Read the model definition and answer for the solid it produces. Units are mm, in the model's axes. A direction names the side the tool comes from. Coordinates: 2 decimals unless noted, no trailing zeros. Write each loop counter-clockwise with the first axis right and the second up, starting at its lowest first coordinate (ties: lowest second). Pieces come first, ordered by that corner, then holes.
(1) Section D-D on x = 0 is taken. Write down the section's boundary in (y, z).
(2) Section A-A on z = 0 is taken. Write down the section's boundary in (x, y), then the cut area to 3 significant figures.
(3) Find the intervals of material crossed by probe 1 along Z at (x, y) = (0, 63); probe 2 along X at (y, z) = (62.65, 0); probe 3 along Y at (x, z) = (-22.5, -23), in increasing order.
(4) Section C-C on y = 28.5 is taken. Write down the section's boundary in (x, z).
(5) Given pin 1 (0.9 mm diameter, centred on y = 60, z = 13.5, fed in from +X); pin 2 (2 mm diameter, centred on x = 43.5, y = 10, fed in from +Z); pin 3 (8 mm diameter, centred on y = 44, z = 1, fed in from -X); pin 4 (8 mm diameter, centred on y = 35.5, z = -1, fed in from +X), each flat-ended and moving along its own axis, determine where each tip first touches the part or whether it passes through.
(6) Which of the six approach directions +Z, -Z, +X, -X, +Y, -Y give full straight-line access (tool end or side, diameter ignored) to faces 1 (the cylindrical face through (2.79, 63.54, -77.95)), 2 (the flat face through (60.661, 12.325, 36.594)), 3 (the flat face through (-30, 40, 56)), 4 (the cylindrical face through (32.66, 58.71, -30.74))?
(7) The mould has two halves that part along X. Classify faces 5 (the flat face through (-67, 0, 43)), 6 (the cylindrical face through (-62, 11, -58)), 7 (the flat face through (-30, 40, -55)): +X half, -X half, draft (parallel to the pull), parting line (faces both ways), or undercut.
(8) Section B-B on y = 19 is taken. Write down the section's boundary in (x, z).
from build123d import *

# Parameters (mm, degrees)
BOSS_EXTRUDE1_DEPTH     = 66
CUT_EXTRUDE3_DEPTH      = 25
CUT_EXTRUDE3_DEPTH_BACK = 10
FILLET1_R               = 4
FILLET3_R               = 9
SKETCH4_W               = 60
SKETCH4_H               = 150
CUT_EXTRUDE4_DEPTH      = 33
CUT_EXTRUDE5_DEPTH      = 5
CUT_EXTRUDE6_DEPTH      = 132.030530793
FILLET5_R               = 3
FILLET6_R               = 5
FILLET7_R               = 3
SKETCH7_R               = 1.5
CUT_EXTRUDE7_DEPTH      = 198.739948877
SKETCH11_R              = 3
CUT_EXTRUDE10_DEPTH     = 210.0771447
SKETCH8_R               = 1.5
CUT_EXTRUDE8_DEPTH      = 205.670582053
SKETCH10_R              = 3
CUT_EXTRUDE9_DEPTH      = 216.914390172
FILLET10_R              = 5


with BuildPart() as part:
    # Sketch3 → Boss-Extrude1 (new body)
    with BuildSketch(Plane(origin=(0, 0, 0), x_dir=(1, 0, 0), z_dir=(0, 1, 0))):
        with BuildLine():
            Line((-46.032597146, -75), (46.032597146, -75))
            ThreePointArc((46.032597146, -75), (0, 88), (-46.032597146, -75))
        make_face()
    extrude(amount=BOSS_EXTRUDE1_DEPTH)

    # Sketch2 → Cut-Extrude3 (cut, two sides: drawn at the far end of the back side and taken through both)
    with BuildSketch(Plane(origin=(0, 0, 0), x_dir=(1, 0, 0), z_dir=(0, 1, 0)).offset(-CUT_EXTRUDE3_DEPTH_BACK)):
        with BuildLine():
            Line((68.882903046, 31.406243643), (31.406243643, 68.882903046))
            Line((31.406243643, 68.882903046), (40.598631798, 78.075291201))
            ThreePointArc((40.598631798, 78.075291201), (0, 88), (-40.598631798, 78.075291201))
            Line((-40.598631798, 78.075291201), (-31.406243643, 68.882903046))
            Line((-31.406243643, 68.882903046), (-68.882903046, 31.406243643))
            Line((-68.882903046, 31.406243643), (-78.075291201, 40.598631798))
            ThreePointArc((-78.075291201, 40.598631798), (-87.22877857, 11.624981252), (-85.982636075, -18.734628196))
            Line((-85.982636075, -18.734628196), (-74.724305826, -12.234628196))
            Line((-74.724305826, -12.234628196), (-47.724305826, -59))
            Line((-47.724305826, -59), (-47.724305826, -73.935043338))
            ThreePointArc((-47.724305826, -73.935043338), (-46.881475519, -74.472325418), (-46.032597146, -75))
            ThreePointArc((-46.032597146, -75), (0, -88), (46.032597146, -75))
            ThreePointArc((46.032597146, -75), (46.881475519, -74.472325418), (47.724305826, -73.935043338))
            Line((47.724305826, -73.935043338), (47.724305826, -59))
            Line((47.724305826, -59), (74.724305826, -12.234628196))
            Line((74.724305826, -12.234628196), (85.982636075, -18.734628196))
            ThreePointArc((85.982636075, -18.734628196), (87.49420545, -9.421465529), (88, 0))
            ThreePointArc((88, 0), (85.482821741, 20.897061687), (78.075291201, 40.598631798))
            Line((78.075291201, 40.598631798), (68.882903046, 31.406243643))
        make_face()
    extrude(amount=CUT_EXTRUDE3_DEPTH + CUT_EXTRUDE3_DEPTH_BACK, mode=Mode.SUBTRACT)

    # Fillet1
    fillet1_edges = [part.edges().sort_by_distance(p)[0] for p in [
        (74.724305826, 12.5, 12.234628196),
        (68.882903046, 12.5, -31.406243643),
        (31.406243643, 12.5, -68.882903046),
        (-31.406243643, 12.5, -68.882903046),
        (-68.882903046, 12.5, -31.406243643),
        (-74.724305826, 12.5, 12.234628196),
    ]]
    fillet(fillet1_edges, radius=FILLET1_R)

    # Fillet3
    fillet3_edges = [part.edges().sort_by_distance(p)[0] for p in [
        (47.724305826, 12.5, 59),
        (-47.724305826, 12.5, 59),
    ]]
    fillet(fillet3_edges, radius=FILLET3_R)

    # Sketch4 → Cut-Extrude4 (cut)
    with BuildSketch(Plane.XZ.offset(-25)):
        Rectangle(SKETCH4_W, SKETCH4_H)
        with BuildLine():
            Line((30, -75), (-30, -75))
            ThreePointArc((-30, -75), (0, -80.777472107), (30, -75))
        make_face()
    extrude(amount=-CUT_EXTRUDE4_DEPTH, mode=Mode.SUBTRACT)

    # Sketch5 → Cut-Extrude5 (cut)
    with BuildSketch(Plane(origin=(0, 66, 0), x_dir=(1, 0, 0), z_dir=(0, 1, 0))):
        with BuildLine():
            Line((-43.116122275, -65), (43.116122275, -65))
            ThreePointArc((43.116122275, -65), (0, 78), (-43.116122275, -65))
        make_face()
    extrude(amount=-CUT_EXTRUDE5_DEPTH, mode=Mode.SUBTRACT)

    # Sketch6 → Cut-Extrude6 (cut, through all)
    with BuildSketch(Plane.XZ.offset(-25)):
        Polygon((30, 35), (50, 15), (50, -15), (30, -35), align=None)
        Polygon((-50, -15), (-30, -35), (-30, 35), (-50, 15), align=None)
    extrude(amount=-CUT_EXTRUDE6_DEPTH, mode=Mode.SUBTRACT)

    # Fillet5
    fillet5_edges = [part.edges().sort_by_distance(p)[0] for p in [
        (30, 59.5, -35),
        (30, 59.5, 35),
        (-30, 59.5, 35),
        (-30, 59.5, -35),
    ]]
    fillet(fillet5_edges, radius=FILLET5_R)

    # Fillet6
    fillet6_edges = [part.edges().sort_by_distance(p)[0] for p in [
        (30, 41.5, -35),
        (30, 41.5, 35),
        (50, 43, 15),
        (50, 43, -15),
        (-30, 41.5, 35),
        (-50, 43, -15),
        (-50, 43, 15),
        (-30, 41.5, -35),
    ]]
    fillet(fillet6_edges, radius=FILLET6_R)

    # Fillet7
    fillet7_edges = [part.edges().sort_by_distance(p)[0] for p in [
        (-30, 41.5, -75),
        (30, 58, -56.035533906),
        (0, 58, -80.777472107),
        (30, 41.5, -75),
        (-30, 58, -56.035533906),
        (-33.292893219, 58, 31.707106781),
        (33.292893219, 58, -31.707106781),
        (33.292893219, 58, 31.707106781),
        (30, 58, 56.035533906),
        (-30, 58, 56.035533906),
        (-33.292893219, 58, -31.707106781),
        (30.380602337, 58, -35.15765065),
        (30.380602337, 58, 35.15765065),
        (-30.380602337, 58, 35.15765065),
        (-30.380602337, 58, -35.15765065),
    ]]
    fillet(fillet7_edges, radius=FILLET7_R)

    # Sketch7 → Cut-Extrude7 (cut, through all)
    with BuildSketch(Plane(origin=(50.144573344, 0, -50.144573344), x_dir=(0.7071067811865472, 0, 0.7071067811865478), z_dir=(-0.7071067811865478, 0, 0.7071067811865472))):
        with Locations((0, 10)):
            Circle(SKETCH7_R)
    cut_extrude7 = extrude(amount=-CUT_EXTRUDE7_DEPTH, mode=Mode.SUBTRACT)

    # Sketch11 → Cut-Extrude10 (cut, through all)
    with BuildSketch(Plane(origin=(58.629854718, 0, -58.629854718), x_dir=(0.7071067811865472, 0, 0.7071067811865478), z_dir=(-0.7071067811865478, 0, 0.7071067811865472))):
        with Locations((0, 10)):
            Circle(SKETCH11_R)
    cut_extrude10 = extrude(amount=-CUT_EXTRUDE10_DEPTH, mode=Mode.SUBTRACT)

    # Sketch8 → Cut-Extrude8 (cut, through all)
    with BuildSketch(Plane(origin=(61.340978781, 0, 35.415230611), x_dir=(-0.5000000000000003, 0, 0.8660254037844386), z_dir=(-0.8660254037844385, 0, -0.5000000000000002))):
        with Locations((0, 10)):
            Circle(SKETCH8_R)
    cut_extrude8 = extrude(amount=-CUT_EXTRUDE8_DEPTH, mode=Mode.SUBTRACT)

    # Sketch10 → Cut-Extrude9 (cut, through all)
    with BuildSketch(Plane(origin=(71.733283626, 0, 41.415230611), x_dir=(-0.5000000000000003, 0, 0.8660254037844386), z_dir=(-0.8660254037844385, 0, -0.5000000000000002))):
        with Locations((0, 10)):
            Circle(SKETCH10_R)
    cut_extrude9 = extrude(amount=-CUT_EXTRUDE9_DEPTH, mode=Mode.SUBTRACT)

    # Mirror1: Cut-Extrude7, Cut-Extrude10, Cut-Extrude8, Cut-Extrude9 across plane
    add(cut_extrude7.mirror(Plane(origin=(0, 0, 0), x_dir=(0, 0, 1), z_dir=(1, 0, 0))), mode=Mode.SUBTRACT)
    add(cut_extrude10.mirror(Plane(origin=(0, 0, 0), x_dir=(0, 0, 1), z_dir=(1, 0, 0))), mode=Mode.SUBTRACT)
    add(cut_extrude8.mirror(Plane(origin=(0, 0, 0), x_dir=(0, 0, 1), z_dir=(1, 0, 0))), mode=Mode.SUBTRACT)
    add(cut_extrude9.mirror(Plane(origin=(0, 0, 0), x_dir=(0, 0, 1), z_dir=(1, 0, 0))), mode=Mode.SUBTRACT)

    # Fillet10
    fillet10_edges = [part.edges().sort_by_distance(p)[0] for p in [
        (46.032597146, 45.5, 75),
        (-46.032597146, 45.5, 75),
    ]]
    fillet(fillet10_edges, radius=FILLET10_R)


solid = part.part
Response:
1. outline: (25, -88) - (66, -88) - (66, -78) - (61, -78) - (61, 65) - (66, 65) - (66, 75) - (58, 75) - (58, -77.78) arc R3 cw to (55, -80.78) - (25, -80.78) - close
2. outline: (-88, 25) - (-50, 25) - (-50, 61) - (-78, 61) - (-78, 66) - (-88, 66) - close; (-30, 58) - (30, 58) - (30, 61) - (-30, 61) - close; (50, 25) - (88, 25) - (88, 66) - (78, 66) - (78, 61) - (50, 61) - close
2. area: 3,020 mm2
3. probe 1: z = -88 to -78, 65 to 75
3. probe 2: x = -88 to -78, 78 to 88
3. probe 3: y = 58 to 61
4. outline: (-50, -12.93) - (-50, 12.93) arc R5 cw to (-48.54, 16.46) - (-31.46, 33.54) arc R5 ccw to (-30, 37.07) - (-30, 75) - (-44.6, 75) arc R5 ccw to (-47.28, 74.22) arc R88 ccw (long way) to (47.28, 74.22) arc R5 ccw to (44.6, 75) - (30, 75) - (30, 37.07) arc R5 ccw to (31.46, 33.54) - (48.54, 16.46) arc R5 cw to (50, 12.93) - (50, -12.93) arc R5 cw to (48.54, -16.46) - (31.46, -33.54) arc R5 ccw to (30, -37.07) - (30, -72.94) arc R3 cw to (28.04, -75.75) arc R80.78 cw to (-28.04, -75.75) arc R3 cw to (-30, -72.94) - (-30, -37.07) arc R5 ccw to (-31.46, -33.54) - (-48.54, -16.46) arc R5 cw to start
5. pin 1: stops at x = 87.03
5. pin 2: stops at z = -55.79
5. pin 3: stops at x = -88
5. pin 4: stops at x = 88
6. face 1: +Y
6. face 2: -Y
6. face 3: +Z, -Y
6. face 4: +Y, -Y
7. face 5: draft
7. face 6: undercut
7. face 7: undercut
8. outline: (-85.98, 18.73) - (-78.19, 14.23) arc R4 ccw to (-72.72, 15.7) - (-48.93, 56.91) arc R9 ccw to (-47.72, 61.41) - (-47.72, 73.94) arc R88 ccw to start; (-78.08, -40.6) arc R88 ccw to (-40.6, -78.08) - (-34.23, -71.71) arc R4 ccw to (-34.23, -66.05) - (-66.05, -34.23) arc R4 ccw to (-71.71, -34.23) - close; (34.23, -71.71) - (40.6, -78.08) arc R88 ccw to (78.08, -40.6) - (71.71, -34.23) arc R4 ccw to (66.05, -34.23) - (34.23, -66.05) arc R4 ccw to start; (47.72, 61.41) arc R9 ccw to (48.93, 56.91) - (72.72, 15.7) arc R4 ccw to (78.19, 14.23) - (85.98, 18.73) arc R88 ccw to (47.72, 73.94) - close
